Here's how the part is built. I have some questions about the finished solid (model axes, mm). A direction names the side the tool comes from. Coordinates: 2 decimals unless noted, no trailing zeros. Loops run counter-clockwise (first coordinate to the right, second up) from the corner with the lowest first, then second, coordinate; pieces in that order, holes last. Notation, with made-up numbers: M 41.5,30.25 L 55.5,30.25 A22 ccw 55.5,50.25 Z; hole C 30,8 d1. An arc over 180 degrees is marked long. Use one line per item in the form item = value. Start each with the question number.
(1) Imagine slicing it at D-D, the plane z = 3.35. Please give me the cut outline in (x, y), and give its area (3 significant figures).
(2) Will these pins go through, and if not, where does the flat tip stop? P1, Ø2, axis at x = 40.5, z = 2.5, coming from the -Y side; P2, Ø2, axis at x = 7, z = 2.5, coming from the +Y side; P3, Ø2, axis at x = 32.5, z = 2, coming from the -Y side (3 decimals); P4, Ø2.5, axis at x = 41.25, y = 32.25, coming from the +Z side.
(3) On a 3-axis mill with a long thin cutter (end or side, diameter ignored), from which of +Z, -Z, +X, -X, +Y, -Y can I reach the whole of each face in a straight line? I mean faces 4 (the flat face through (39, 0, 2)), 5 (the flat face through (15.514, 38.232, 1.972)), 6 (the flat face through (6, 0, 2)). Say none if no direction works.
(4) Thinking about a two-plate mould opening in X: for faces 1 (the flat face through (36.4, 22, 2)), 2 (the flat face through (31.986, -1.267, 1.972)), 3 (the flat face through (39, 37, 2)), which applies, +X half, -X half, draft (parallel to the pull), parting line (faces both ways), or undercut?
(5) Imagine slicing it at B-B, the plane x = 41.25. Please give me the cut outline in (y, z).
(6) Imagine slicing it at C-C, the plane x = 30. Please give me the cut outline in (y, z).
(7) Imagine slicing it at A-A, the plane y = 21. Please give me the cut outline in (x, z), and give its area (3 significant figures).
(8) Please list where these lines run through material, in increasing order: L1, parallel to Y at x = 4.25, z = 1.6; L2, parallel to Y at x = 10.5, z = 2.5; L3, parallel to X at y = 28, z = 1.05.
```python
from build123d import *

# Parameters (mm, degrees)
SKETCH1_W              = 45.5
SKETCH1_H              = 37
BASIS_DEPTH            = 4
SKETCH6_W              = 27.3
SKETCH6_H              = 15.480915405
SHOW_ONLY_SCREEN_DEPTH = 10.04
SKETCH11_R             = 1.6
CUT_EXTRUDE10_DEPTH    = 4


with BuildPart() as part:
    # Sketch1 → Basis (new body)
    with BuildSketch(Plane.XY):
        with Locations((22.75, 18.5)):
            Rectangle(SKETCH1_W, SKETCH1_H)
        Polygon((14.5, 39.5), (12.5, 37), (16.5, 37), align=None)
        Polygon((31, 39.5), (29, 37), (33, 37), align=None)
        Polygon((16.5, 0), (12.5, 0), (14.5, -2.5), align=None)
        Polygon((33, 0), (29, 0), (31, -2.5), align=None)
    extrude(amount=BASIS_DEPTH)

    # Sketch6 → Show only screen (cut)
    with BuildSketch(Plane.XY.offset(4)):
        with Locations((22.75, 22.399542298)):
            Rectangle(SKETCH6_W, SKETCH6_H)
    extrude(amount=-SHOW_ONLY_SCREEN_DEPTH, mode=Mode.SUBTRACT)

    # Sketch11 → Cut-Extrude10 (cut)
    with BuildSketch(Plane(origin=(0, 0, 0), x_dir=(-1, 0, 0), z_dir=(0, 0, -1))):
        with Locations((-41.25, 32.252592082)):
            Circle(SKETCH11_R)
        with Locations((-4.25, 32.252592082)):
            Circle(SKETCH11_R)
        with Locations((-4.25, 12.252592082)):
            Circle(SKETCH11_R)
        with Locations((-41.25, 12.252592082)):
            Circle(SKETCH11_R)
    extrude(amount=-CUT_EXTRUDE10_DEPTH, mode=Mode.SUBTRACT)


solid = part.part
```
Answer:
q1.outline = M 0,0 L 12.5,0 L 14.5,-2.5 L 16.5,0 L 29,0 L 31,-2.5 L 33,0 L 45.5,0 L 45.5,37 L 33,37 L 31,39.5 L 29,37 L 16.5,37 L 14.5,39.5 L 12.5,37 L 0,37 Z; hole C 4.25,12.25 d3.2; hole C 4.25,32.25 d3.2; hole M 9.1,14.66 L 36.4,14.66 L 36.4,30.14 L 9.1,30.14 Z; hole C 41.25,12.25 d3.2; hole C 41.25,32.25 d3.2
q1.area = 1,250 mm²
q2.P1 = 0
q2.P2 = 37
q2.P3 = -1.875
q2.P4 = through
q3.face_4 = +Z, -Z, +X, -Y
q3.face_5 = +Z, -Z, +Y
q3.face_6 = +Z, -Z, -X, -Y
q4.face_1 = undercut
q4.face_2 = +X half
q4.face_3 = draft
q5.outline = M 0,0 L 10.65,0 L 10.65,4 L 0,4 Z; M 13.85,0 L 30.65,0 L 30.65,4 L 13.85,4 Z; M 33.85,0 L 37,0 L 37,4 L 33.85,4 Z
q6.outline = M -1.25,0 L 14.66,0 L 14.66,4 L -1.25,4 Z; M 30.14,0 L 38.25,0 L 38.25,4 L 30.14,4 Z
q7.outline = M 0,0 L 9.1,0 L 9.1,4 L 0,4 Z; M 36.4,0 L 45.5,0 L 45.5,4 L 36.4,4 Z
q7.area = 72.8 mm²
q8.L1 = 0 to 10.65, 13.85 to 30.65, 33.85 to 37
q8.L2 = 0 to 14.66, 30.14 to 37
q8.L3 = 0 to 9.1, 36.4 to 45.5
